```python
from build123d import *

# Parameters (mm, degrees)
F1_DEPTH  = 1.5875
F2_W      = 125.4125
F2_H      = 107.95
F3_DEPTH  = 1.5875
F4_W      = 127
F4_H      = 127
F4_W_2    = 125.4125
F5_DEPTH  = 1.5875
F7_DEPTH  = 1.5875
F9_DEPTH  = 127
F11_DEPTH = 127
F13_DEPTH = 711.201
F14_R     = 12.7
F15_DEPTH = 25.4
F16_R     = 14.2875
F16_R_2   = 12.7
F17_DEPTH = 25.4
F18_W     = 123.825
F18_H     = 25.4
F19_DEPTH = 1.5875


with BuildPart() as f1:
    # F0 (on Front) → F1 (new body)
    with BuildSketch(Plane.XZ):
        Polygon((355.6, 120.65), (-355.6, 120.65), (-355.6, 12.7), (139.7, -6.35), (355.6, -6.35), align=None)
    extrude(amount=-F1_DEPTH)

    # F2 (on face) → F3 (join)
    with BuildSketch(Plane(origin=(-355.6, 0, 0), x_dir=(0, -1, 0), z_dir=(-1, 0, 0))):
        with Locations((-64.29375, 66.675)):
            Rectangle(F2_W, F2_H)
    extrude(amount=-F3_DEPTH)

    # F4 (on face) → F5 (join)
    with BuildSketch(Plane.YZ.offset(355.6)):
        with Locations((63.5, 57.15)):
            Rectangle(F4_W, F4_H)
        with Locations((64.29375, 57.15)):
            Rectangle(F4_W_2, F4_H)
    extrude(amount=-F5_DEPTH)

    # F6 (on face) → F7 (join)
    with BuildSketch(Plane(origin=(0, 127, 0), x_dir=(-1, 0, 0), z_dir=(0, 1, 0))):
        Polygon((355.6, 12.7), (355.6, 120.65), (-355.6, 120.65), (-355.6, -6.35), (-139.7, -6.35), align=None)
    extrude(amount=-F7_DEPTH)

    # F8 (on face) → F9 (join)
    with BuildSketch(Plane.XZ):
        Polygon((-355.6, 14.2875), (-355.6, 12.7), (139.7, -6.35), (355.6, -6.35), (355.6, -4.7625), (139.7, -4.7625), align=None)
    extrude(amount=-F9_DEPTH)

    # F10 (on face) → F11 (join)
    with BuildSketch(Plane.XZ):
        Polygon((90.4875, 120.65), (88.9, 120.65), (88.9, -4.396154), (90.4875, -4.457212), align=None)
    extrude(amount=-F11_DEPTH)

    # F12 (on face) → F13 (cut, through all)
    with BuildSketch(Plane.YZ.offset(355.6)):
        with BuildLine():
            Line((50.8, 120.65), (50.8, 82.55))
            ThreePointArc((50.8, 82.55), (63.5, 69.85), (76.2, 82.55))
            Line((76.2, 82.55), (76.2, 120.65))
            Line((76.2, 120.65), (63.5, 120.65))
            Line((63.5, 120.65), (50.8, 120.65))
        make_face()
    extrude(amount=-F13_DEPTH, mode=Mode.SUBTRACT)

    # F14 (on face) → F15 (cut)
    with BuildSketch(Plane.XY.offset(-4.7625)):
        with Locations((163.5125, 63.5)):
            Circle(F14_R)
    extrude(amount=-F15_DEPTH, mode=Mode.SUBTRACT)

    # F16 (on face) → F17 (join)
    with BuildSketch(Plane(origin=(0, 0, -6.35), x_dir=(1, 0, 0), z_dir=(0, 0, -1))):
        with Locations((163.5125, -63.5)):
            Circle(F16_R)
        with Locations((163.5125, -63.5)):
            Circle(F16_R_2, mode=Mode.SUBTRACT)
    extrude(amount=F17_DEPTH)

    # F18 (on face) → F19 (cut)
    with BuildSketch(Plane.YZ.offset(90.4875)):
        with Locations((63.5, 9.830288)):
            Rectangle(F18_W, F18_H)
    extrude(amount=-F19_DEPTH, mode=Mode.SUBTRACT)


solid = f1.part
```
The model under review builds one solid part; all positions refer to its coordinate system, in mm. A direction names the side the tool comes from. Coordinates: 2 decimals unless noted, no trailing zeros. Write each loop counter-clockwise with the first axis right and the second up, starting at its lowest first coordinate (ties: lowest second). Pieces come first, ordered by that corner, then holes. Notation, with made-up numbers: (26.25, 87.25) - (42.25, 87.25) arc R8 cw to (42.25, 98.25) - close; hole circle Ø3 at (42, 77.5). An arc over 180 degrees is marked (long way). Answer in a Markdown table with one row per item. Add a question column.
Q1. Consider section A-A on y = 63.5. Give the number of separate pieces and of enclosed holes in the cut face, then the cut area to 3 significant figures.
Q2. To check wall thickness, follow line 1 along X through (y, z) = (10.5, 61); line 2 along Y through (x, z) = (38, 9); line 3 along X through (y, z) = (63.5, -22.25) (1 decimal). State the ranges of each line that lie inside material, in increasing order. Write a range as from..to.
Q3. For faces 1 (the face through (88.9, 63, 61)), 2 (the face through (177.14, 59.21, -18.87)), 3 (the face through (-355.6, 64, 67)), list the 3-axis set-ups (+Z, -Z, +X, -X, +Y, -Y) from which the entire face can be reached by the end or side of a thin tool; tool diameter is ignored.
Q4. Consider section B-B on z = 45. Give the boundary of the cut face in (x, y), then the cut area to 3 significant figures.
Q5. Clearance check with flat-ended pins moving along their axes: pin 1 (1 mm diameter, centred on x = -116.5, y = 36, fed in from -Z); pin 2 (5 mm diameter, centred on x = 197.5, y = 50.5, fed in from +Z); pin 3 (2 mm diameter, centred on x = -229, z = 31, fed in from -Y); pin 4 (1 mm diameter, centred on x = -100, y = 17.5, fed in from +Z). State where each tip first meets the part, or that it passes through.
Q6. Consider section C-C on y = 37.5. Give the boundary of the cut face in (x, z).
Q7. Consider section D-D on x = 242. Give the boundary of the cut face in (y, z).
Q8. Draft analysis for pull direction X (two halves, no side actions). For faces 4 (the face through (-104.48, 64.39, 3.04)), 5 (the face through (355.6, 63, 56)), 6 (the face through (248, 63, -4.762)), state which applies: +X half, -X half, draft (parallel to the pull), parting line (faces both ways), or undercut.
Answers below:
| question | item | result |
|---|---|---|
| 1 | separate pieces | 3 |
| 1 | enclosed holes | 0 |
| 1 | area | 1,450 mm² |
| 2 | line 1 | -355.6..-354.01, 88.9..90.49, 354.01..355.6 |
| 2 | line 2 | 0..1.59, 125.41..127 |
| 2 | line 3 | 149.2..150.8, 176.2..177.8 |
| 3 | face 1 | +Z |
| 3 | face 2 | -Z |
| 3 | face 3 | +Z, -Z, -X, +Y, -Y |
| 4 | outline | (-355.6, 0) - (355.6, 0) - (355.6, 127) - (-355.6, 127) - close; hole (-354.01, 1.59) - (88.9, 1.59) - (88.9, 125.41) - (-354.01, 125.41) - close; hole (90.49, 1.59) - (354.01, 1.59) - (354.01, 125.41) - (90.49, 125.41) - close |
| 4 | area | 2,850 mm² |
| 5 | pin 1 | z = 3.48 |
| 5 | pin 2 | z = -4.76 |
| 5 | pin 3 | y = 0 |
| 5 | pin 4 | z = 4.48 |
| 6 | outline | (-355.6, 12.7) - (139.7, -6.35) - (355.6, -6.35) - (355.6, 120.65) - (354.01, 120.65) - (354.01, -4.76) - (139.7, -4.76) - (90.49, -2.87) - (88.9, -2.87) - (88.9, -2.81) - (-354.01, 14.23) - (-354.01, 120.65) - (-355.6, 120.65) - close; (88.9, 22.53) - (90.49, 22.53) - (90.49, 120.65) - (88.9, 120.65) - close |
| 7 | outline | (0, -6.35) - (127, -6.35) - (127, 120.65) - (125.41, 120.65) - (125.41, -4.76) - (1.59, -4.76) - (1.59, 120.65) - (0, 120.65) - close |
| 8 | face 4 | -X half |
| 8 | face 5 | +X half |
| 8 | face 6 | undercut |
